Autodesk Inventor part; units mm, degrees
ref_plane "YZ Plane" through (0, 0, 0) normal (1, 0, 0) x (0, 1, 0)
ref_plane "XZ Plane" through (0, 0, 0) normal (0, 1, 0) x (-1, 0, 0)
ref_plane "XY Plane" through (0, 0, 0) normal (0, 0, 1) x (1, 0, 0)
sketch "Sketch1" plane through (0, 0, 0) normal (0, 0, 1) x (1, 0, 0)
  line L0 (0, 0) -> (279.4, 0)
  line L1 (279.4, 0) -> (279.4, 25.4)
  line L2 (279.4, 25.4) -> (0, 25.4)
  line L3 (0, 25.4) -> (0, 0)
  dimension "d0" = 279.4
  dimension "d1" = 25.4
extrude "Extrusion1" add sketch "Sketch1" along normal blind 25.4
sketch "Sketch4" plane through (0, 0, 25.4) normal (0, 0, 1) x (1, 0, 0)
  circle A0 centre (12.7, 12.7) radius 2.3813
  line L0 (0, 0) -> (279.4, 0)
  line L1 (0, 25.4) -> (0, 0)
  circle A1 centre (38.1, 12.7) radius 2.3813
  circle A2 centre (63.5, 12.7) radius 2.3813
  circle A3 centre (88.9, 12.7) radius 2.3813
  circle A4 centre (114.3, 12.7) radius 2.3813
  circle A5 centre (139.7, 12.7) radius 2.3813
  circle A6 centre (165.1, 12.7) radius 2.3813
  circle A7 centre (190.5, 12.7) radius 2.3813
  circle A8 centre (215.9, 12.7) radius 2.3813
  circle A9 centre (241.3, 12.7) radius 2.3813
  circle A10 centre (266.7, 12.7) radius 2.3813
  circle A11 centre (292.1, 12.7) radius 2.3813
  circle A12 centre (317.5, 12.7) radius 2.3813
  circle A13 centre (63.5, 12.7) radius 9.525
  circle A14 centre (5.08, 6.35) radius 3.175
  dimension "d17" = 4.7625
  dimension "d18" = 12.7
  dimension "d19" = 12.7
  dimension "d22" = 25.4
  dimension "d37" = 19.05
  dimension "d46" = 6.35
  dimension "d48" = 6.35
  dimension "d49" = 58.42
extrude "Extrusion4" cut sketch "Sketch4" against normal blind 25.4 contours A0 | A1 | A2 | A3 | A4 | A5 | A6 | A7 | A8 | A9 | A10 | A11 | A12 | A13 | A14
sketch "Sketch6" plane through (0, 25.4, 0) normal (0, 1, 0) x (1, 0, 0)
  line L0 (19.05, -22.225) -> (0, -22.225)
  line L1 (0, -22.225) -> (0, -3.175)
  line L2 (0, -3.175) -> (19.05, -3.175)
  line L3 (19.05, -3.175) -> (19.05, -22.225)
  line L4 (279.4, 0) -> (279.4, -25.4)
  line L5 (279.4, -25.4) -> (0, -25.4)
  line L6 (279.4, 0) -> (0, 0)
  line L7 (0, 0) -> (0, -25.4)
  dimension "d38" = 19.05
  dimension "d41" = 3.175
  dimension "d42" = 3.175
  dimension "d45" = 0
extrude "Extrusion6" cut sketch "Sketch6" against normal blind 25.4 contours L0 L1 L2 L3
sketch "Sketch7" plane through (0, 25.4, 0) normal (0, 1, 0) x (1, 0, 0)
  circle A0 centre (266.7, -18.9992) radius 2.0701
  circle A1 centre (266.7, -6.2992) radius 2.0701
  line L0 (279.4, 0) -> (279.4, -25.4)
  line L1 (279.4, 0) -> (0, 0)
  line L2 (279.4, -25.4) -> (0, -25.4)
  dimension "d50" = 4.1402
  dimension "d51" = 4.1402
  dimension "d52" = 12.7
  dimension "d53" = 12.7
  dimension "d54" = 12.7
  dimension "d58" = 6.4008
extrude "Extrusion7" cut sketch "Sketch7" against normal blind 25.4
equation "\"d42\" = d41"
equation "\"d51\" = d50"
equation "\"d53\" = d54"
properties part number "RobotArm Arm"
Could you check a few things on this model? Use its own coordinates, in mm. A direction names the side the tool comes from. Give positions to 0.01 mm unless a question says otherwise; leave off trailing zeros. Loops run counter-clockwise (first coordinate to the right, second up) from the corner with the lowest first, then second, coordinate; pieces in that order, holes last. Notation, with made-up numbers: (-24.75, 13.25) -> (25.25, 13.25) arc R26 cw to (25.25, 49.25) -> close; hole circle Ø3 at (35.5, 75). An arc over 180 degrees is marked (long way). Return JSON: item names as keys, results as strings.
Item 1: We'd pull the mould along X, two halves only. Please class faces 3 (the cylindrical face through (14.97, 13.42, 23.83)), 4 (the flat face through (279.4, 13, 13)), 5 (the flat face through (9, 13, 3.175)): +X half, -X half, draft (parallel to the pull), parting line (faces both ways), or undercut.
Geometry results:
{"face 3": "undercut", "face 4": "+X half", "face 5": "draft"}
Item 2: If we section it at B-B on y = 18.25: List the corners of the cut face in (x, z) for me (3 decimals).
Geometry results:
{"outline": "(0, 0) -> (55.759, 0) -> (55.759, 25.4) -> (0, 25.4) -> (0, 22.225) -> (19.05, 22.225) -> (19.05, 3.175) -> (0, 3.175) -> close; (71.241, 0) -> (279.4, 0) -> (279.4, 25.4) -> (71.241, 25.4) -> close; hole circle Ø4.14 at (266.7, 6.299); hole circle Ø4.14 at (266.7, 18.999)"}
Item 3: I'm going to push flat-ended pins straight in: pin 1 (12 mm diameter, centred on x = 242, y = 5.5, fed in from -Z); pin 2 (1.5 mm diameter, centred on y = 15.5, z = 5.5, fed in from -X). Where does each tip first touch, or does it pass through?
Geometry results:
{"pin 1": "stops at z = 0", "pin 2": "stops at x = 19.05"}
Item 4: If we section it at C-C on z = 12: Count the separate pieces of the cut face and the enclosed holes in it, plus the area to 3 significant figures.
Geometry results:
{"separate pieces": "1", "enclosed holes": "10", "area": "6,170 mm²"}
Item 5: If we section it at D-D on x = 165.1: List the corners of the cut face in (y, z) for me, plus the area to 3 significant figures.
Geometry results:
{"outline": "(0, 0) -> (10.32, 0) -> (10.32, 25.4) -> (0, 25.4) -> close; (15.08, 0) -> (25.4, 0) -> (25.4, 25.4) -> (15.08, 25.4) -> close", "area": "524 mm²"}
Item 6: I need wall thicknesses on L1, parallel to Z at x = 18, y = 5.75 (3 decimals); L2, parallel to Z at x = 266.7, y = 6.5; L3, parallel to Y at x = 190.5, z = 5.75. Which ranges of each line are inside material? Lowest first, please. Write a range as from..to.
Geometry results:
{"L1": "z = 0..3.175, 22.225..25.4", "L2": "z = 0..4.23, 8.37..16.93, 21.07..25.4", "L3": "y = 0..10.32, 15.08..25.4"}
Item 7: Which directions (+Z, -Z, +X, -X, +Y, -Y) give clear straight access to the entire face, cutting with the end or side of a thin tool? Please do faces 1 (the flat face through (19.05, 13, 13)), 2 (the flat face through (138, 10, 0)).
Geometry results:
{"face 1": "-X, +Y, -Y", "face 2": "-Z, +X, -X, +Y, -Y"}
Item 8: If we section it at A-A on x = 5.08: List the corners of the cut face in (y, z) for me (3 decimals), plus the area to 3 significant figures.
Geometry results:
{"outline": "(0, 0) -> (3.175, 0) -> (3.175, 3.175) -> (0, 3.175) -> close; (0, 22.225) -> (3.175, 22.225) -> (3.175, 25.4) -> (0, 25.4) -> close; (9.525, 0) -> (25.4, 0) -> (25.4, 3.175) -> (9.525, 3.175) -> close; (9.525, 22.225) -> (25.4, 22.225) -> (25.4, 25.4) -> (9.525, 25.4) -> close", "area": "121 mm²"}
